```python
from build123d import *

# Parameters (mm, degrees)
SKETCH1_R           = 45
BOSS_EXTRUDE1_DEPTH = 3
SKETCH2_W           = 10
SKETCH2_H           = 40
BOSS_EXTRUDE2_DEPTH = 65
CUT_EXTRUDE1_REACH  = 114.979
SKETCH3_R           = 5


with BuildPart() as part:
    # Sketch1 → Boss-Extrude1 (new body)
    with BuildSketch(Plane(origin=(0, 0, 0), x_dir=(1, 0, 0), z_dir=(0, 1, 0))):
        with Locations(Location((0, 0, 0), (0, 0, 270))):
            Circle(SKETCH1_R)
    extrude(amount=BOSS_EXTRUDE1_DEPTH)

    # Sketch2 → Boss-Extrude2 (add)
    with BuildSketch(Plane(origin=(0, 3, 0), x_dir=(1, 0, 0), z_dir=(0, 1, 0))):
        with Locations((-28.200807343, 0)):
            Rectangle(SKETCH2_W, SKETCH2_H)
        with Locations((28.200807343, 0)):
            Rectangle(SKETCH2_W, SKETCH2_H)
    extrude(amount=BOSS_EXTRUDE2_DEPTH)

    # Cut-Extrude1: up to this face of the body (flat: up to its plane)
    cut_extrude1_end = Plane(part.part.faces().sort_by_distance((33.200807343, 35.5, 0))[0])
    # Sketch3 → Cut-Extrude1 (cut, up to the picked face)
    with BuildSketch(Plane.ZY.offset(33.200807343), mode=Mode.PRIVATE) as cut_extrude1_sk1:
        with Locations((0, 58)):
            Circle(SKETCH3_R)
    cut_extrude1_tool1 = split(extrude(cut_extrude1_sk1.sketch, amount=-CUT_EXTRUDE1_REACH, mode=Mode.PRIVATE), bisect_by=cut_extrude1_end, keep=Keep.BOTH, mode=Mode.PRIVATE)
    add(cut_extrude1_tool1.solids().sort_by(Axis((-33.200807, 58, 0), (1, 0, 0)))[0], mode=Mode.SUBTRACT)


solid = part.part
```
For this review, take the finished solid that the model builds, in its own axes (mm). A direction names the side the tool comes from. Coordinates: 2 decimals unless noted, no trailing zeros. Order: outer loops, then holes, each group sorted by start corner. A loop starts at its lowest first (then second) coordinate and runs counter-clockwise, first axis right, second up. Notation, with made-up numbers: (47, 28) -> (102, 28) arc R29 ccw to (102, 55) -> close; hole circle Ø5 at (-12.75, -28.75). An arc over 180 degrees is marked (long way). Use CSV: the item, a comma, the result in double quotes. Start each with the question number.
Item 1: We need section D-D, the plane z = 16. Give the boundary of the cut face in (x, y), then the cut area to 3 significant figures.
Item 2: Wall thickness on probe 1 along X at (y, z) = (25.5, -8); probe 2 along Y at (x, z) = (26.75, 0); probe 3 along Y at (x, z) = (2, -17.5): over which ranges is each line inside the solid? List them lowest first.
Item 3: We need section A-A, the plane y = 12.5. Give the boundary of the cut face in (x, z), then the cut area to 3 significant figures.
Item 4: We need section B-B, the plane z = 0. Give the boundary of the cut face in (x, y).
Item 5: Draft analysis for pull direction Z (two halves, no side actions). For faces 1 (the face through (28, 35, 20)), 2 (the face through (28, 35, -20)), 3 (the face through (-33.201, 35, 0)), 4 (the face through (-28.271, 62.957, -0.651)), state which applies: pulls with the +Z half, pulls with the -Z half, needs draft (parallel to the pull), parting line crosses it, or undercut.
Item 6: We need section C-C, the plane y = 58. Give the boundary of the cut face in (x, z), then the cut area to 3 significant figures.
Item 7: Insertion check: pin 1 (12 mm diameter, centred on y = 17.5, z = -21.5, fed in from -X); pin 2 (5 mm diameter, centred on x = -28, y = 46, fed in from -Z); pin 3 (12 mm diameter, centred on x = -27.5, y = 29.5, fed in from +Z). Each pin has a flat end and moves straight along its axis. Give the tip position at first contact, or say it passes through.
Item 8: For faces 5 (the face through (-28, 35, -20)), 6 (the face through (23.201, 35, 0)), 7 (the face through (33.201, 35, 0)), list the 3-axis set-ups (+Z, -Z, +X, -X, +Y, -Y) from which the entire face can be reached by the end or side of a thin tool; tool diameter is ignored.
Derived:
1,outline,"(-42.06, 0) -> (42.06, 0) -> (42.06, 3) -> (33.2, 3) -> (33.2, 68) -> (23.2, 68) -> (23.2, 3) -> (-23.2, 3) -> (-23.2, 68) -> (-33.2, 68) -> (-33.2, 3) -> (-42.06, 3) -> close"
1,area,"1,550 mm^2"
2,probe 1,"x = -33.2 to -23.2, 23.2 to 33.2"
2,probe 2,"y = 0 to 53, 63 to 68"
2,probe 3,"y = 0 to 3"
3,outline,"(-33.2, -20) -> (-23.2, -20) -> (-23.2, 20) -> (-33.2, 20) -> close; (23.2, -20) -> (33.2, -20) -> (33.2, 20) -> (23.2, 20) -> close"
3,area,"800 mm^2"
4,outline,"(-45, 0) -> (45, 0) -> (45, 3) -> (33.2, 3) -> (33.2, 53) -> (23.2, 53) -> (23.2, 3) -> (-23.2, 3) -> (-23.2, 53) -> (-33.2, 53) -> (-33.2, 3) -> (-45, 3) -> close; (-33.2, 63) -> (-23.2, 63) -> (-23.2, 68) -> (-33.2, 68) -> close; (23.2, 63) -> (33.2, 63) -> (33.2, 68) -> (23.2, 68) -> close"
5,face 1,"pulls with the +Z half"
5,face 2,"pulls with the -Z half"
5,face 3,"needs draft"
5,face 4,"undercut"
6,outline,"(-33.2, -20) -> (-23.2, -20) -> (-23.2, -5) -> (-33.2, -5) -> close; (-33.2, 5) -> (-23.2, 5) -> (-23.2, 20) -> (-33.2, 20) -> close; (23.2, -20) -> (33.2, -20) -> (33.2, -5) -> (23.2, -5) -> close; (23.2, 5) -> (33.2, 5) -> (33.2, 20) -> (23.2, 20) -> close"
6,area,"600 mm^2"
7,pin 1,"stops at x = -33.2"
7,pin 2,"stops at z = -20"
7,pin 3,"stops at z = 20"
8,face 5,"-Z, +X, -X, +Y"
8,face 6,"+Z, -Z, +Y"
8,face 7,"+Z, -Z, +X, +Y"
